from build123d import *

# Parameters (mm, degrees)
BOSS_EXTRUDE1_DEPTH = 1.2
FILLET1_R           = 5
FILLET2_R           = 0.8


with BuildPart() as part:
    # Sketch1 → Boss-Extrude1 (new body)
    with BuildSketch(Plane.XY):
        with BuildLine():
            Line((-10.5, 0), (-12.5, -2))
            Line((-12.5, -2), (-12, -12))
            Line((-12, -12), (-12.5, -14))
            Line((-12.5, -14), (-14.5, -14))
            Line((-14.5, -14), (-14.5, 3))
            Line((-14.5, 3), (-12.5, 3))
            Line((-12.5, 3), (12.5, 3))
            Line((12.5, 3), (14.5, 3))
            Line((14.5, 3), (14.5, -14))
            Line((14.5, -14), (12.5, -14))
            Line((12.5, -14), (12, -12))
            Line((12, -12), (12.5, -2))
            Line((12.5, -2), (10.5, 0))
            Line((10.5, 0), (8, 0))
            Line((8, 0), (8, -12))
            Line((8, -12), (3.5, -12))
            Line((3.5, -12), (3.5, -6))
            ThreePointArc((3.5, -6), (0, -2.5), (-3.5, -6))
            Line((-3.5, -6), (-3.5, -12))
            Line((-3.5, -12), (-8, -12))
            Line((-8, -12), (-8, 0))
            Line((-8, 0), (-10.5, 0))
        make_face()
    extrude(amount=BOSS_EXTRUDE1_DEPTH)

    # Fillet1
    fillet1_edges = [part.edges().sort_by_distance(p)[0] for p in [
        (-12, -12, 0.6),
        (12, -12, 0.6),
    ]]
    fillet(fillet1_edges, radius=FILLET1_R)

    # Fillet2
    fillet2_edges = [part.edges().sort_by_distance(p)[0] for p in [
        (-12.5, -14, 0.6),
        (-14.5, -14, 0.6),
        (-14.5, 3, 0.6),
        (14.5, 3, 0.6),
        (14.5, -14, 0.6),
        (12.5, -14, 0.6),
        (8, -12, 0.6),
        (3.5, -12, 0.6),
        (-3.5, -12, 0.6),
        (-8, -12, 0.6),
    ]]
    fillet(fillet2_edges, radius=FILLET2_R)


solid = part.part
Work out the finished part from the listing and answer in its coordinate system (mm). A direction names the side the tool comes from. Coordinates: 2 decimals unless noted, no trailing zeros. Loops run counter-clockwise (first coordinate to the right, second up) from the corner with the lowest first, then second, coordinate; pieces in that order, holes last. Notation, with made-up numbers: M -23.75,57.5 L 24.25,57.5 A29 cw 24.25,95.5 Z; hole C -33.5,85.5 d3. An arc over 180 degrees is marked long. Answer in a Markdown table with one row per item. Add a question column.
1. The mould has two halves that part along Y. Classify faces 4 (the flat face through (-12.27, -6.56, 0.59)), 5 (the flat face through (3.5, -9, 1)), 6 (the cylindrical face through (14.26, 2.77, 0.61)), 7 (the flat face through (-6, -12, 1)): pulls with the +Y half, pulls with the -Y half, needs draft (parallel to the pull), parting line crosses it, or undercut.
2. A tool of negligible diameter and unlimited length cuts with its end or side. For faces 1 (the flat face through (0, 3, 1)), 2 (the cylindrical face through (-12.054, -11.984, 0.608)), 3 (the cylindrical face through (3.73, -11.76, 0.61)), from which of +Z, -Z, +X, -X, +Y, -Y can it reach the whole face along a straight path? Write none if from no direction.
3. Find section A-A, the plane y = -1. Write down the section's boundary in (x, z).
4. Consider L1, parallel to X at y = -7.5, z = 0.15 (3 decimals); L2, parallel to X at y = -4, z = 0.1; L3, parallel to Y at x = -8.25, z = 0.35. Determine where each line is inside the solid, lowest interval first.
5. Find section D-D, the plane x = 0. Write down the section's boundary in (y, z).
6. Flat-ended cylindrical pins translate along their axes: P1, Ø0.6, axis at x = 6, z = 1, coming from the -Y side; P2, Ø0.6, axis at x = 8.5, z = 0.5, coming from the -Y side. Find the tip coordinate at first contact, or state that the pin passes through.
7. Find section B-B, the plane y = -8. Write down the section's boundary in (x, z), then the cut area to 3 significant figures.
Reported:
| question | item | result |
|---|---|---|
| 1 | face 4 | undercut |
| 1 | face 5 | needs draft |
| 1 | face 6 | pulls with the +Y half |
| 1 | face 7 | pulls with the -Y half |
| 2 | face 1 | +Z, -Z, +X, -X, +Y |
| 2 | face 2 | +Z, -Z |
| 2 | face 3 | +Z, -Z, -Y |
| 3 | outline | M -14.5,0 L -11.5,0 L -11.5,1.2 L -14.5,1.2 Z; M -8,0 L 8,0 L 8,1.2 L -8,1.2 Z; M 11.5,0 L 14.5,0 L 14.5,1.2 L 11.5,1.2 Z |
| 4 | L1 | x = -14.5 to -12.225, -8 to -3.5, 3.5 to 8, 12.225 to 14.5 |
| 4 | L2 | x = -14.5 to -12.4, -8 to -2.87, 2.87 to 8, 12.4 to 14.5 |
| 4 | L3 | y = 0 to 3 |
| 5 | outline | M -2.5,0 L 3,0 L 3,1.2 L -2.5,1.2 Z |
| 6 | P1 | stops at y = -12 |
| 6 | P2 | stops at y = 0 |
| 7 | outline | M -14.5,0 L -12.2,0 L -12.2,1.2 L -14.5,1.2 Z; M -8,0 L -3.5,0 L -3.5,1.2 L -8,1.2 Z; M 3.5,0 L 8,0 L 8,1.2 L 3.5,1.2 Z; M 12.2,0 L 14.5,0 L 14.5,1.2 L 12.2,1.2 Z |
| 7 | area | 16.3 mm^2 |
